from build123d import *

# Parameters (mm, degrees)
F0_R     = 6.35
F1_DEPTH = 63.5
F3_DEPTH = 12.7
F4_R     = 3.175
F5_DEPTH = 25.4
F6_R     = 2.54
F7_DEPTH = 25.4


with BuildPart() as f1:
    # F0 (on Front) → F1 (new body)
    with BuildSketch(Plane.XZ):
        Circle(F0_R)
    extrude(amount=F1_DEPTH)

    # F2 (on face) → F3 (cut)
    with BuildSketch(Plane.XZ.offset(63.5)):
        with BuildLine():
            Line((0, 5.08), (3.81, 5.08))
            ThreePointArc((3.81, 5.08), (0, 6.35), (-3.81, 5.08))
            Line((-3.81, 5.08), (0, 5.08))
        make_face()
        with BuildLine():
            ThreePointArc((-3.81, -5.08), (0, -6.35), (3.81, -5.08))
            Line((3.81, -5.08), (-3.81, -5.08))
        make_face()
        with BuildLine():
            ThreePointArc((3.81, -5.08), (5.6796126628, -2.8398063314), (6.35, 0))
            ThreePointArc((6.35, 0), (5.6796126628, 2.8398063314), (3.81, 5.08))
            Line((3.81, 5.08), (3.81, -5.08))
        make_face()
        with BuildLine():
            Line((-3.81, -5.08), (-3.81, 5.08))
            ThreePointArc((-3.81, 5.08), (-6.35, 0), (-3.81, -5.08))
        make_face()
    extrude(amount=-F3_DEPTH, mode=Mode.SUBTRACT)

    # F4 (on face) → F5 (cut)
    with BuildSketch(Plane.YZ.offset(3.81)):
        with Locations((-57.15, 0)):
            Circle(F4_R)
    extrude(amount=-F5_DEPTH, mode=Mode.SUBTRACT)

    # F6 (on face) → F7 (cut)
    with BuildSketch(Plane(origin=(0, 0, 0), x_dir=(-1, 0, 0), z_dir=(0, 1, 0))):
        Circle(F6_R)
    extrude(amount=-F7_DEPTH, mode=Mode.SUBTRACT)


solid = f1.part
Verification items for the finished model (mm, model axes). A direction names the side the tool comes from. Give positions to 0.01 mm unless a question says otherwise; leave off trailing zeros. Loops run counter-clockwise (first coordinate to the right, second up) from the corner with the lowest first, then second, coordinate; pieces in that order, holes last.
1) Sectioned sample at D-D, the plane y = -5. Enter the section's corners in (x, z), then the cut area to 3 significant figures.
2) Set-up check for faces 1 (the flat face through (5, -50.8, 0)), 2 (the flat face through (-3.81, -57.2, -3.5)), 3 (the flat face through (0, -25.4, 0)), 4 (the flat face through (0, -57, 5.08)), 5 (the flat face through (0, -57, -5.08)): record each of +Z, -Z, +X, -X, +Y, -Y from which the full face is reachable in a straight line by a thin tool's end or side.
3) Depth check by flat-ended pin: pin 1 Ø4 at (x, z) = (-0.5, 0.5) entering from +Y; pin 2 Ø1 at (y, z) = (-38, -4.5) entering from +X; pin 3 Ø2.5 at (x, y) = (0, -58.5) entering from -Z; pin 4 Ø5 at (y, z) = (-55, 1) entering from +X. Enter the tip coordinate at first touch or a pass-through.
4) Sectioned sample at B-B, the plane y = -57.15. Enter the section's corners in (x, z) (3 decimals).
5) Sectioned sample at C-C, the plane z = 1. Enter the section's corners in (x, y).
6) Draft check along X on faces 6 (the cylindrical face through (0.33, -12.52, 2.52)), 7 (the flat face through (3, 0, 0)), 8 (the cylindrical face through (-1.38, -25.04, -6.2)). Enter one of: pulls with the +X half, pulls with the -X half, needs draft (parallel to the pull), parting line crosses it, or undercut.
7) Sectioned sample at A-A, the plane x = 0. Enter the section's corners in (y, z) (3 decimals), then the cut area to 3 significant figures.
8) Thickness scan on line 1 along Z through (x, y) = (0, -7); line 2 along Y through (x, z) = (2.75, 0.25); line 3 along Z through (x, y) = (-0.75, -57.15) (3 decimals). Record the ranges inside material, lowest first.
Answers:
1. outline: circle Ø12.7 at (0, 0); hole circle Ø5.08 at (0, 0)
1. area: 106 mm2
2. face 1: +Z, -Z, +X, -Y
2. face 2: +Z, -Z, -X, -Y
2. face 3: +Y
2. face 4: +Z, +X, -X, -Y
2. face 5: -Z, +X, -X, -Y
3. pin 1: stops at y = 0
3. pin 2: stops at x = 4.93
3. pin 3: stops at z = -5.08
3. pin 4: stops at x = 3.81
4. outline: (-3.81, -5.08) - (3.81, -5.08) - (3.81, -3.175) - (-3.81, -3.175) - close; (-3.81, 3.175) - (3.81, 3.175) - (3.81, 5.08) - (-3.81, 5.08) - close
5. outline: (-6.27, -50.8) - (-3.81, -50.8) - (-3.81, -54.14) - (3.81, -54.14) - (3.81, -50.8) - (6.27, -50.8) - (6.27, 0) - (2.33, 0) - (2.33, -25.4) - (-2.33, -25.4) - (-2.33, 0) - (-6.27, 0) - close; (-3.81, -63.5) - (3.81, -63.5) - (3.81, -60.16) - (-3.81, -60.16) - close
6. face 6: undercut
6. face 7: needs draft
6. face 8: parting line crosses it
7. outline: (-63.5, -5.08) - (-50.8, -5.08) - (-50.8, -6.35) - (0, -6.35) - (0, -2.54) - (-25.4, -2.54) - (-25.4, 2.54) - (0, 2.54) - (0, 6.35) - (-50.8, 6.35) - (-50.8, 5.08) - (-63.5, 5.08) - close; hole circle Ø6.35 at (-57.15, 0)
7. area: 613 mm2
8. line 1: z = -6.35 to -2.54, 2.54 to 6.35
8. line 2: y = -63.5 to -60.32, -53.98 to 0
8. line 3: z = -5.08 to -3.175, 3.175 to 5.08
